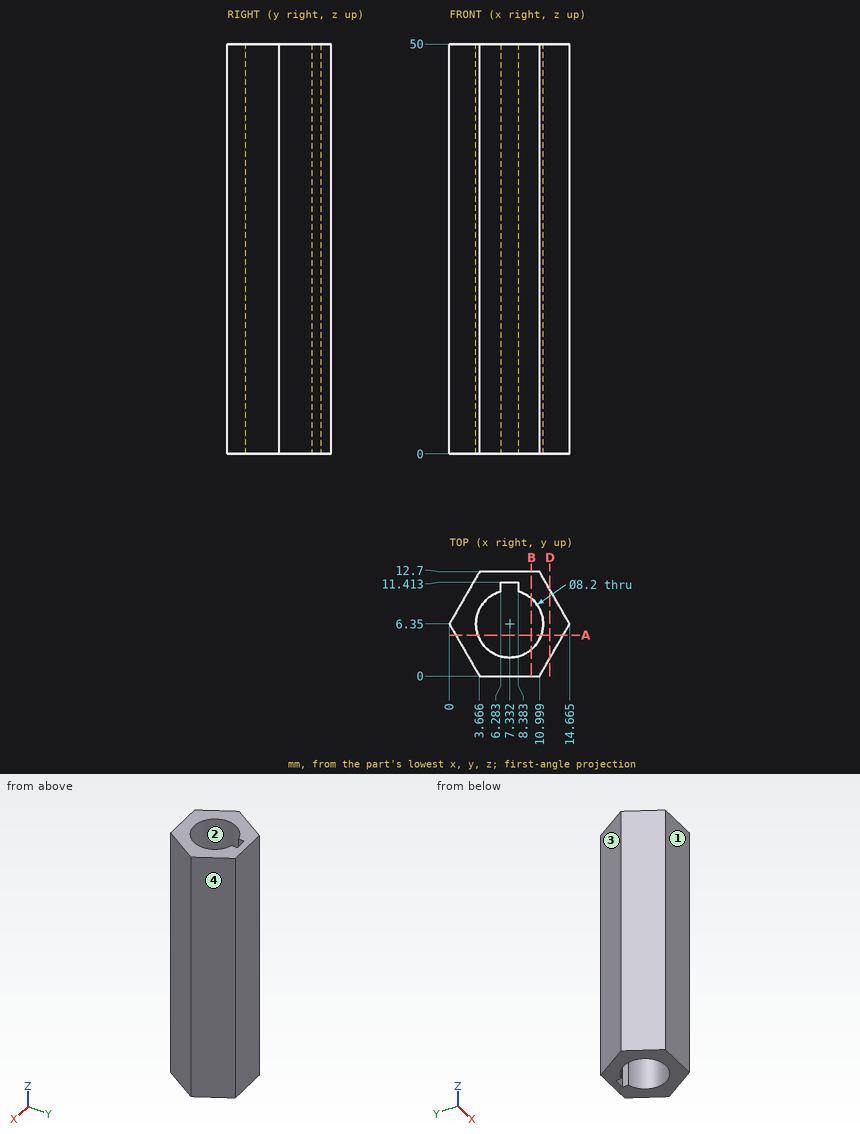
For this review, use the dimensioned drawing (mm, ordinates from the lowest corner) and the shaded views. Coordinates: 2 decimals unless noted, no trailing zeros. Loops run counter-clockwise (first coordinate to the right, second up) from the corner with the lowest first, then second, coordinate; pieces in that order, holes last. Notation, with made-up numbers: (28, 8) -> (68, 8) arc R14 ccw to (68, 13) -> close; hole circle Ø2 at (76.5, -17.75). An arc over 180 degrees is marked (long way). Use a Markdown table: item, result. Add a question column.
1. To check wall thickness, follow line 1 (X direction, y = 6.35, z = 30.5) (1 decimal); line 2 (Y direction, x = 7.5, z = 32); line 3 (Y direction, x = 6, z = 29.5). State the ranges of each line that lie inside material, in increasing order.
2. Draft analysis for pull direction X (two halves, no side actions). For the marked faces 1, 2, 3 and 4, state which applies: pulls with the +X half, pulls with the -X half, needs draft (parallel to the pull), parting line crosses it, or undercut.
3. Add section B-B on x = 10. Write out the cut boundary in (y, z).
4. Add section D-D on x = 12.25. Write out the cut boundary in (y, z), plus the area to 3 significant figures.
5. Clearance check with flat-ended pins moving along their axes: pin 1 Ø5 at (x, y) = (7.33, 6.35) entering from -Z; pin 2 Ø4 at (y, z) = (9.5, 40) entering from +X; pin 3 Ø0.6 at (y, z) = (11, 31) entering from -X; pin 4 Ø4 at (y, z) = (4, 38) entering from -X. State where each tip first meets the part, or that it passes through.
6. Add section A-A on y = 5. Write out the cut boundary in (x, z) (1 decimal), plus the area to 3 significant figures.
Returned:
| question | item | result |
|---|---|---|
| 1 | line 1 | x = 0 to 3.2, 11.4 to 14.7 |
| 1 | line 2 | y = 0 to 2.25, 11.41 to 12.7 |
| 1 | line 3 | y = 0 to 2.47, 10.23 to 12.7 |
| 2 | face 1 | needs draft |
| 2 | face 2 | undercut |
| 2 | face 3 | pulls with the -X half |
| 2 | face 4 | pulls with the +X half |
| 3 | outline | (0, 0) -> (3.24, 0) -> (3.24, 50) -> (0, 50) -> close; (9.46, 0) -> (12.7, 0) -> (12.7, 50) -> (9.46, 50) -> close |
| 4 | outline | (2.17, 0) -> (10.53, 0) -> (10.53, 50) -> (2.17, 50) -> close |
| 4 | area | 418 mm² |
| 5 | pin 1 | passes through |
| 5 | pin 2 | stops at x = 14 |
| 5 | pin 3 | stops at x = 2.51 |
| 5 | pin 4 | stops at x = 0.2 |
| 6 | outline | (0.8, 0) -> (3.5, 0) -> (3.5, 50) -> (0.8, 50) -> close; (11.2, 0) -> (13.9, 0) -> (13.9, 50) -> (11.2, 50) -> close |
| 6 | area | 268 mm² |
